Read the model definition and answer for the solid it produces. Units are mm, in the model's axes. Coordinates: 2 decimals unless noted, no trailing zeros. Order: outer loops, then holes, each group sorted by start corner. A loop starts at its lowest first (then second) coordinate and runs counter-clockwise, first axis right, second up. Notation, with made-up numbers: (-22.5, 86) - (26.5, 86) arc R21 cw to (26.5, 106) - close; hole circle Ø5 at (77, 75.25). An arc over 180 degrees is marked (long way). Answer as a JSON object with one key per item and string values. Group by question number.
Autodesk Fusion 360 part; units mm, degrees
sketch "Sketch4" plane through (0, 0, 0) normal (0, 1, 0) x (1, 0, 0)
  circle A0 centre (0, 0) radius 16.375
  dimension "d2" = 32.75
extrude "Extrude1" add sketch "Sketch4" along normal blind 0.35
sketch "Sketch5" plane through (0, 0.35, 0) normal (0, 1, 0) x (-1, 0, 0)
  circle A0 centre (0, 0) radius 16.375
  circle A1 centre (0, 0) radius 0.85
  line L0 (-3.45, -0.875) -> (-10.45, -0.875)
  line L1 (-10.45, -0.875) -> (-10.45, 0.875)
  line L2 (-10.45, 0.875) -> (-3.45, 0.875)
  line L3 (-3.45, 0.875) -> (-3.45, -0.875)
  dimension "d11" = 1.7
  dimension "d12" = 7
  dimension "d14" = 1.75
  dimension "d15" = 3.45
  dimension "d16" = 0.875
extrude "Extrude2" cut sketch "Sketch5" against normal through all contours A1 | L0 L1 L2 L3
sketch "Sketch7" plane through (0, 0.35, 0) normal (0, 1, 0) x (-1, 0, 0)
  circle A0 centre (0, 0) radius 0.85
  line L0 (-3.45, 0.875) -> (-3.45, -0.875)
  line L1 (-3.45, -0.875) -> (-10.45, -0.875)
  line L2 (-10.45, -0.875) -> (-10.45, 0.875)
  line L3 (-10.45, 0.875) -> (-3.45, 0.875)
  circle A1 centre (0, 0) radius 16.375
  line L4 (0.375, 12.5) -> (-0.375, 12.5)
  line L5 (-0.375, 12.5) -> (-0.375, 14.5)
  line L6 (-0.375, 14.5) -> (0.375, 14.5)
  line L7 (0.375, 14.5) -> (0.375, 12.5)
  circle A2 centre (0, 0) radius 15.5
  line L8 (-6.5748, 10.6378) -> (-7.5748, 12.3699)
  line L9 (-6.9252, 12.7449) -> (-5.9252, 11.0128)
  line L10 (-5.9252, 11.0128) -> (-6.5748, 10.6378)
  line L11 (-7.5748, 12.3699) -> (-6.9252, 12.7449)
  line L12 (-11.0128, 5.9252) -> (-12.7449, 6.9252)
  line L13 (-12.3699, 7.5748) -> (-10.6378, 6.5748)
  line L14 (-10.6378, 6.5748) -> (-11.0128, 5.9252)
  line L15 (-12.7449, 6.9252) -> (-12.3699, 7.5748)
  line L16 (-10.6378, -6.5748) -> (-12.3699, -7.5748)
  line L17 (-12.7449, -6.9252) -> (-11.0128, -5.9252)
  line L18 (-11.0128, -5.9252) -> (-10.6378, -6.5748)
  line L19 (-12.3699, -7.5748) -> (-12.7449, -6.9252)
  line L20 (-5.9252, -11.0128) -> (-6.9252, -12.7449)
  line L21 (-7.5748, -12.3699) -> (-6.5748, -10.6378)
  line L22 (-6.5748, -10.6378) -> (-5.9252, -11.0128)
  line L23 (-6.9252, -12.7449) -> (-7.5748, -12.3699)
  line L24 (6.5748, -10.6378) -> (7.5748, -12.3699)
  line L25 (6.9252, -12.7449) -> (5.9252, -11.0128)
  line L26 (5.9252, -11.0128) -> (6.5748, -10.6378)
  line L27 (7.5748, -12.3699) -> (6.9252, -12.7449)
  line L28 (11.0128, -5.9252) -> (12.7449, -6.9252)
  line L29 (12.3699, -7.5748) -> (10.6378, -6.5748)
  line L30 (10.6378, -6.5748) -> (11.0128, -5.9252)
  line L31 (12.7449, -6.9252) -> (12.3699, -7.5748)
  line L32 (10.6378, 6.5748) -> (12.3699, 7.5748)
  line L33 (12.7449, 6.9252) -> (11.0128, 5.9252)
  line L34 (11.0128, 5.9252) -> (10.6378, 6.5748)
  line L35 (12.3699, 7.5748) -> (12.7449, 6.9252)
  line L36 (5.9252, 11.0128) -> (6.9252, 12.7449)
  line L37 (7.5748, 12.3699) -> (6.5748, 10.6378)
  line L38 (6.5748, 10.6378) -> (5.9252, 11.0128)
  line L39 (6.9252, 12.7449) -> (7.5748, 12.3699)
  line L40 (0.75, -14.5) -> (-0.75, -14.5)
  line L41 (-0.75, -14.5) -> (0, -11.75)
  line L42 (0, -11.75) -> (0.75, -14.5)
  line L43 (0, -14.5) -> (0, -11.75)
  line L44 (-12.5, -0.375) -> (-14.5, -0.375)
  line L45 (-14.5, 0.375) -> (-12.5, 0.375)
  line L46 (-12.5, 0.375) -> (-12.5, -0.375)
  line L47 (-14.5, -0.375) -> (-14.5, 0.375)
  line L48 (12.5, 0.375) -> (14.5, 0.375)
  line L49 (14.5, -0.375) -> (12.5, -0.375)
  line L50 (12.5, -0.375) -> (12.5, 0.375)
  line L51 (14.5, 0.375) -> (14.5, -0.375)
  dimension "d20" = 0.75
  dimension "d21" = 2
  dimension "d24" = 31
  dimension "d26" = 0.375
  dimension "d31" = 2.75
  dimension "d32" = 1.5
  dimension "d33" = 0.75
  dimension "d34" = 14.5
  dimension "d35" = 14.5
sketch "Sketch8" plane through (0, 0.35, 0) normal (0, 1, 0) x (-1, 0, 0)
  circle A0 centre (0, 0) radius 0.85
  line L0 (-3.45, 0.875) -> (-3.45, -0.875)
  line L1 (-3.45, -0.875) -> (-10.45, -0.875)
  line L2 (-10.45, -0.875) -> (-10.45, 0.875)
  line L3 (-10.45, 0.875) -> (-3.45, 0.875)
  circle A1 centre (0, 0) radius 16.375
  line L4 (-5.4637, -8.2785) -> (-5.7091, -8.2785) construction
  line L5 (-5.7091, -8.2785) -> (-5.7091, -10.7785) construction
  line L6 (-5.7091, -10.7785) -> (-5.4637, -10.7785) construction
  line L7 (-5.4637, -10.7785) -> (-5.4637, -8.2785) construction
  line L8 (-9.0419, -4.7) -> (-9.8, -4.7) construction
  line L9 (-9.8, -4.7) -> (-9.8, -7.2) construction
  line L10 (-9.8, -7.2) -> (-9.0419, -7.2) construction
  line L11 (-9.0419, -7.2) -> (-9.0419, -4.7) construction
  line L12 (-11.1719, 1.0124) -> (-11.9349, 1.0124) construction
  line L13 (-11.9349, 1.0124) -> (-11.9349, -1.4876) construction
  line L14 (-11.9349, -1.4876) -> (-11.1719, -1.4876) construction
  line L15 (-11.1719, -1.4876) -> (-11.1719, 1.0124) construction
  line L16 (7.2613, -3.0997) -> (-7.3506, -3.0997) construction
  line L17 (-7.3506, -3.0997) -> (-7.3506, -6.0997) construction
  line L18 (-7.3506, -6.0997) -> (7.2613, -6.0997) construction
  line L19 (7.2613, -6.0997) -> (7.2613, -3.0997) construction
  line L20 (5.6532, -8.2) -> (4.9, -8.2) construction
  line L21 (4.9, -8.2) -> (4.9, -10.7) construction
  line L22 (4.9, -10.7) -> (5.6532, -10.7) construction
  line L23 (5.6532, -10.7) -> (5.6532, -8.2) construction
  line L24 (9.9968, -4.559) -> (8.654, -4.559) construction
  line L25 (8.654, -4.559) -> (8.654, -7.059) construction
  line L26 (8.654, -7.059) -> (9.9968, -7.059) construction
  line L27 (9.9968, -7.059) -> (9.9968, -4.559) construction
  line L28 (-9, 6.5) -> (-9.8447, 6.5) construction
  line L29 (-9.8447, 6.5) -> (-9.8447, 4) construction
  line L30 (-9.8447, 4) -> (-9, 4) construction
  line L31 (-9, 4) -> (-9, 6.5) construction
  line L32 (-5.2603, 10.2723) -> (-6, 10.2723) construction
  line L33 (-6, 10.2723) -> (-6, 7.7723) construction
  line L34 (-6, 7.7723) -> (-5.2603, 7.7723) construction
  line L35 (-5.2603, 7.7723) -> (-5.2603, 10.2723) construction
  line L36 (0.375, 11.567) -> (-0.3818, 11.567) construction
  line L37 (-0.3818, 11.567) -> (-0.3818, 9.067) construction
  line L38 (-0.3818, 9.067) -> (0.375, 9.067) construction
  line L39 (0.375, 9.067) -> (0.375, 11.567) construction
  line L40 (5.7526, 10.3802) -> (4.9958, 10.3802) construction
  line L41 (4.9958, 10.3802) -> (4.9958, 7.8802) construction
  line L42 (4.9958, 7.8802) -> (5.7526, 7.8802) construction
  line L43 (5.7526, 7.8802) -> (5.7526, 10.3802) construction
  line L44 (10, 6.5) -> (9.2249, 6.5) construction
  line L45 (9.2249, 6.5) -> (9.2249, 4) construction
  line L46 (9.2249, 4) -> (10, 4) construction
  line L47 (10, 4) -> (10, 6.5) construction
  line L48 (11.7568, 1) -> (11, 1) construction
  line L49 (11, 1) -> (11, -1.5) construction
  line L50 (11, -1.5) -> (11.7568, -1.5) construction
  line L51 (11.7568, -1.5) -> (11.7568, 1) construction
  line L52 (0.6011, -9.0275) -> (-0.6721, -9.0275) construction
  line L53 (-0.6721, -9.0275) -> (-0.6721, -11.5275) construction
  line L54 (-0.6721, -11.5275) -> (0.6011, -11.5275) construction
  line L55 (0.6011, -11.5275) -> (0.6011, -9.0275) construction
1. Straight lines are drawn through the part: L1, parallel to Z at x = 0, y = 0.25 (3 decimals); L2, parallel to Z at x = 7.5, y = 0.2 (3 decimals); L3, parallel to X at y = 0.25, z = 1.5. For each, find the intervals that lie inside material, in ascending order.
2. A cutting plane is placed at B-B on x = 0. Write down the section's boundary in (y, z) (3 decimals).
3. For a pull along Z with two mould halves and no side action, classify faces 1 (the cylindrical face through (15.62, 0.17, 4.92)), 2 (the cylindrical face through (0.18, 0.18, -0.83)), 3 (the flat face through (0, 0.35, 3)) as pulls with the +Z half, pulls with the -Z half, needs draft (parallel to the pull), parting line crosses it, or undercut.
4. A cutting plane is placed at D-D on x = 7. Write down the section's boundary in (y, z) (3 decimals).
5. A cutting plane is placed at C-C on y = 0.1. Write down the section's boundary in (x, z) (3 decimals), and give its area (3 significant figures).
6. A cutting plane is placed at A-A on z = 0. Write down the section's boundary in (x, y) (3 decimals).
7. Given pin 1 (1.5 mm diameter, centred on x = 0, z = 0, fed in from -Y), flat-ended and moving along its own axis, determine where the tip first touches the part or whether it passes through.
Derived:
{
 "1": {"L1": "z = -16.375 to -0.85, 0.85 to 16.375", "L2": "z = -14.556 to -0.875, 0.875 to 14.556", "L3": "x = -16.31 to 16.31"},
 "2": {"outline": "(0, -16.375) - (0.35, -16.375) - (0.35, -0.85) - (0, -0.85) - close; (0, 0.85) - (0.35, 0.85) - (0.35, 16.375) - (0, 16.375) - close"},
 "3": {"face 1": "parting line crosses it", "face 2": "undercut", "face 3": "needs draft"},
 "4": {"outline": "(0, -14.803) - (0.35, -14.803) - (0.35, -0.875) - (0, -0.875) - close; (0, 0.875) - (0.35, 0.875) - (0.35, 14.803) - (0, 14.803) - close"},
 "5": {"outline": "circle Ø32.75 at (0, 0); hole circle Ø1.7 at (0, 0); hole (3.45, -0.875) - (10.45, -0.875) - (10.45, 0.875) - (3.45, 0.875) - close", "area": "828 mm2"},
 "6": {"outline": "(-16.375, 0) - (-0.85, 0) - (-0.85, 0.35) - (-16.375, 0.35) - close; (0.85, 0) - (3.45, 0) - (3.45, 0.35) - (0.85, 0.35) - close; (10.45, 0) - (16.375, 0) - (16.375, 0.35) - (10.45, 0.35) - close"},
 "7": {"pin 1": "passes through"}
}
